Check sheet for the modelled part. Datum: model origin and axes. Units: mm. Face numbers are marked on the shaded views. A direction names the side the tool comes from. Round coordinates to 2 decimals unless told otherwise and drop trailing zeros. Write each loop counter-clockwise with the first axis right and the second up, starting at its lowest first coordinate (ties: lowest second). Pieces come first, ordered by that corner, then holes. Notation, with made-up numbers: (54.25, -16.5) - (106.25, -16.5) arc R6 ccw to (106.25, -9.5) - close; hole circle Ø8 at (44, 13). An arc over 180 degrees is marked (long way). Answer as a JSON object with one key per item and string values. Group by question number.
Item 1: Thickness scan on line 1 (X direction, y = -5.75, z = 55); line 2 (X direction, y = -2.75, z = 22); line 3 (Z direction, x = 14.5, y = -5.25). Record the ranges inside material, lowest first.
Item 2: Set-up check for the marked faces 5, 6 and 7: record each of +Z, -Z, +X, -X, +Y, -Y from which the full face is reachable in a straight line by a thin tool's end or side.
Item 3: Sectioned sample at D-D on y = -2.25. Count the separate pieces of the cut face and the enclosed holes in it, plus the area to 3 significant figures.
Item 4: Sectioned sample at C-C on y = -9.25. Record the boundary of the cut face in (x, z).
Item 5: Sectioned sample at A-A on x = 35. Record the boundary of the cut face in (y, z).
Item 6: Sectioned sample at B-B on z = 18.5. Record the boundary of the cut face in (x, y).
Item 7: Release check for a two-part mould opening along X. For the marked faces 1, 2, 3 and 4 record: pulls with the +X half, pulls with the -X half, needs draft (parallel to the pull), parting line crosses it, or undercut.
Item 8: Gauge pin test, flat ends, axial feed: P1, Ø1.2, axis at y = -4, z = 53.5, coming from the +X side; P2, Ø3, axis at y = -4.5, z = 53, coming from the +X side; P3, Ø4.5, axis at y = -5.5, z = 54, coming from the +X side. Record the tip position at first contact, or that the pin passes through.
```python
from build123d import *

# Parameters (mm, degrees)
F0_W     = 65
F0_H     = 65
F1_DEPTH = 8
F2_W     = 65
F2_H     = 65
F3_DEPTH = 3
F5_DEPTH = 11.001
F7_DEPTH = 11.001
F9_DEPTH = 8
F10_R    = 1


with BuildPart() as f1:
    # F0 (on Front) → F1 (new body)
    with BuildSketch(Plane.XZ):
        with Locations((28.5, 28)):
            Rectangle(F0_W, F0_H)
        Polygon((12, 0), (0, 0), (0, 56), (12, 56), (12, 52), (15, 52), (15, 56), (27, 56), (27, 52), (30, 52), (30, 56), (42, 56), (42, 52), (45, 52), (45, 56), (57, 56), (57, 0), (45, 0), (45, 4), (42, 4), (42, 0), (30, 0), (30, 4), (27, 4), (27, 0), (15, 0), (15, 4), (12, 4), align=None, mode=Mode.SUBTRACT)
    extrude(amount=F1_DEPTH)

    # F2 (on face) → F3 (join)
    with BuildSketch(Plane.XZ.offset(8)):
        with Locations((28.5, 28)):
            Rectangle(F2_W, F2_H)
        Polygon((12, 4), (12, 0), (0, 0), (0, 56), (12, 56), (12, 52), (15, 52), (15, 56), (27, 56), (27, 52), (30, 52), (30, 56), (42, 56), (42, 52), (45, 52), (45, 56), (57, 56), (57, 0), (45, 0), (45, 4), (42, 4), (42, 0), (30, 0), (30, 4), (27, 4), (27, 0), (15, 0), (15, 4), align=None, mode=Mode.SUBTRACT)
        Polygon((0, 0), (12, 0), (12, 4), (15, 4), (15, 0), (27, 0), (27, 4), (30, 4), (30, 0), (42, 0), (42, 4), (45, 4), (45, 0), (57, 0), (57, 56), (45, 56), (45, 52), (42, 52), (42, 56), (30, 56), (30, 52), (27, 52), (27, 56), (15, 56), (15, 52), (12, 52), (12, 56), (0, 56), align=None)
    extrude(amount=F3_DEPTH)

    # F4 (on face) → F5 (cut, through all)
    with BuildSketch(Plane.XZ.offset(11)):
        with BuildLine():
            Line((9.5, 4), (47.5, 4))
            ThreePointArc((47.5, 4), (51.0355339059, 5.4644660941), (52.5, 9))
            Line((52.5, 9), (52.5, 47))
            ThreePointArc((52.5, 47), (51.0355339059, 50.5355339059), (47.5, 52))
            Line((47.5, 52), (9.5, 52))
            ThreePointArc((9.5, 52), (5.9644660941, 50.5355339059), (4.5, 47))
            Line((4.5, 47), (4.5, 9))
            ThreePointArc((4.5, 9), (5.9644660941, 5.4644660941), (9.5, 4))
        make_face()
    extrude(amount=-F5_DEPTH, mode=Mode.SUBTRACT)

    # F6 (on face) → F7 (cut, through all)
    with BuildSketch(Plane.XZ.offset(11)):
        with BuildLine():
            ThreePointArc((-4, 50.8869504303), (0.3925054478, 56.1074945522), (5.6130495697, 60.5))
            Line((5.6130495697, 60.5), (-4, 60.5))
            Line((-4, 60.5), (-4, 50.8869504303))
        make_face()
        with BuildLine():
            Line((61, 60.5), (51.3869504303, 60.5))
            ThreePointArc((51.3869504303, 60.5), (56.6074945522, 56.1074945522), (61, 50.8869504303))
            Line((61, 50.8869504303), (61, 60.5))
        make_face()
        with BuildLine():
            Line((61, -4.5), (61, 5.1130495697))
            ThreePointArc((61, 5.1130495697), (56.6074945522, -0.1074945522), (51.3869504303, -4.5))
            Line((51.3869504303, -4.5), (61, -4.5))
        make_face()
        with BuildLine():
            ThreePointArc((5.6130495697, -4.5), (0.3925054478, -0.1074945522), (-4, 5.1130495697))
            Line((-4, 5.1130495697), (-4, -4.5))
            Line((-4, -4.5), (5.6130495697, -4.5))
        make_face()
    extrude(amount=-F7_DEPTH, mode=Mode.SUBTRACT)

    # F8 (on face) → F9 (cut)
    with BuildSketch(Plane(origin=(0, 0, 0), x_dir=(-1, 0, 0), z_dir=(0, 1, 0))):
        with BuildLine():
            ThreePointArc((-54.9136378655, 57.7049193689), (-55.6366618004, 59.0201509297), (-55.8869504303, 60.5))
            Line((-55.8869504303, 60.5), (-61, 60.5))
            Line((-61, 60.5), (-62.4552159954, 54.6130084653))
            ThreePointArc((-62.4552159954, 54.6130084653), (-58.7438875569, 54.1901486861), (-56.9998547435, 50.8869504303))
            Line((-56.9998547435, 50.8869504303), (-51.3869504303, 50.8869504303))
            Line((-51.3869504303, 50.8869504303), (-51.3869504303, 56))
            Line((-51.3869504303, 56), (-56.7145795645, 56))
            ThreePointArc((-56.7145795645, 56), (-55.8274078977, 56.866507887), (-54.9136378655, 57.7049193689))
        make_face()
        with BuildLine():
            ThreePointArc((-51.3869504303, 56), (-53.3455388455, 56.4485889594), (-54.9136378655, 57.7049193689))
            ThreePointArc((-54.9136378655, 57.7049193689), (-55.8274078977, 56.866507887), (-56.7145795645, 56))
            Line((-56.7145795645, 56), (-51.3869504303, 56))
        make_face()
        with BuildLine():
            ThreePointArc((-0.2854204355, 56), (-1.1725921023, 56.866507887), (-2.0863621345, 57.7049193689))
            ThreePointArc((-2.0863621345, 57.7049193689), (-3.6544611545, 56.4485889594), (-5.6130495697, 56))
            Line((-5.6130495697, 56), (-0.2854204355, 56))
        make_face()
        with BuildLine():
            ThreePointArc((-1.1130495697, 60.5), (-1.3633381996, 59.0201509297), (-2.0863621345, 57.7049193689))
            ThreePointArc((-2.0863621345, 57.7049193689), (-1.1725921023, 56.866507887), (-0.2854204355, 56))
            Line((-0.2854204355, 56), (-5.6130495697, 56))
            Line((-5.6130495697, 56), (-5.6130495697, 50.8869504303))
            Line((-5.6130495697, 50.8869504303), (-0.0001452565, 50.8869504303))
            ThreePointArc((-0.0001452565, 50.8869504303), (1.7438875569, 54.1901486861), (5.4552159954, 54.6130084653))
            Line((5.4552159954, 54.6130084653), (4, 60.5))
            Line((4, 60.5), (-1.1130495697, 60.5))
        make_face()
        with BuildLine():
            Line((-5.6130495697, 5.1130495697), (-5.6130495697, 0))
            ThreePointArc((-5.6130495697, 0), (-2.4310690543, -1.3180194847), (-1.1130495697, -4.5))
            Line((-1.1130495697, -4.5), (4, -4.5))
            Line((4, -4.5), (5.4552159954, 1.3869915347))
            ThreePointArc((5.4552159954, 1.3869915347), (1.7438875569, 1.8098513139), (-0.0001452565, 5.1130495697))
            Line((-0.0001452565, 5.1130495697), (-5.6130495697, 5.1130495697))
        make_face()
        with BuildLine():
            ThreePointArc((-56.9998547435, 5.1130495697), (-58.7438875569, 1.8098513139), (-62.4552159954, 1.3869915347))
            Line((-62.4552159954, 1.3869915347), (-61, -4.5))
            Line((-61, -4.5), (-55.8869504303, -4.5))
            ThreePointArc((-55.8869504303, -4.5), (-54.5689309457, -1.3180194847), (-51.3869504303, 0))
            Line((-51.3869504303, 0), (-51.3869504303, 5.1130495697))
            Line((-51.3869504303, 5.1130495697), (-56.9998547435, 5.1130495697))
        make_face()
    extrude(amount=-F9_DEPTH, mode=Mode.SUBTRACT)

    # F10
    f10_edges = [f1.edges().sort_by_distance(p)[0] for p in [
        (48.193475, 0, 56),
        (45, 0, 54),
        (53.345539, 0, 56.448589),
        (43.5, 0, 52),
        (42, 0, 54),
        (36, 0, 56),
        (30, 0, 54),
        (28.5, 0, 52),
        (27, 0, 54),
        (21, 0, 56),
        (15, 0, 54),
        (13.5, 0, 52),
        (12, 0, 54),
        (8.806525, 0, 56),
        (57, 0, 28),
        (57.411614, 0, 52.654617),
        (57.411614, 0, 3.345383),
        (53.345539, 0, -0.448589),
        (48.193475, 0, 0),
        (45, 0, 2),
        (43.5, 0, 4),
        (42, 0, 2),
        (36, 0, 0),
        (30, 0, 2),
        (28.5, 0, 4),
        (27, 0, 2),
        (21, 0, 0),
        (15, 0, 2),
        (12, 0, 2),
        (8.806525, 0, 0),
        (0, 0, 28),
        (-0.411614, 0, 3.345383),
        (-0.411614, 0, 52.654617),
        (3.654461, 0, 56.448589),
    ]]
    fillet(f10_edges, radius=F10_R)


solid = f1.part
```
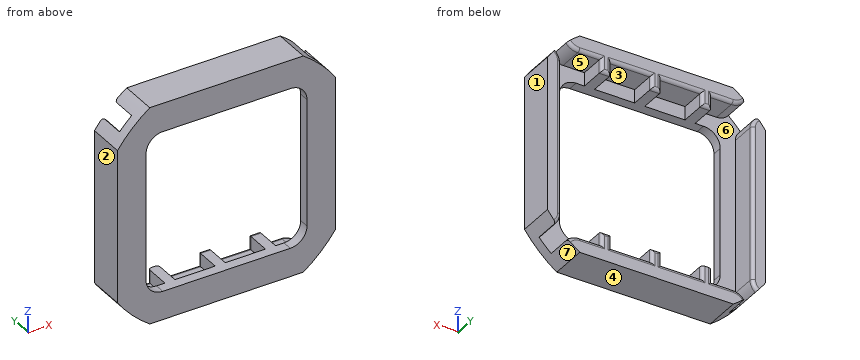
Completed:
{
 "1": {"line 1": "12 to 15, 27 to 30, 42 to 45", "line 2": "-4 to 0, 57 to 61", "line 3": "-4.5 to 4, 52 to 60.5"},
 "2": {"face 5": "+X, +Y", "face 6": "+Y", "face 7": "-Z, +X, +Y, -Y"},
 "3": {"separate pieces": "4", "enclosed holes": "0", "area": "917 mm²"},
 "4": {"outline": "(-4, 5.11) arc R39.75 ccw to (5.61, -4.5) - (51.39, -4.5) arc R39.75 ccw to (61, 5.11) - (61, 50.89) arc R39.75 ccw to (51.39, 60.5) - (5.61, 60.5) arc R39.75 ccw to (-4, 50.89) - close; hole (4.5, 9) arc R5 ccw to (9.5, 4) - (47.5, 4) arc R5 ccw to (52.5, 9) - (52.5, 47) arc R5 ccw to (47.5, 52) - (9.5, 52) arc R5 ccw to (4.5, 47) - close"},
 "5": {"outline": "(-11, -4.5) - (0, -4.5) - (0, -1) arc R1 ccw to (-1, 0) - (-8, 0) - (-8, 4) - (-11, 4) - close; (-11, 52) - (-8, 52) - (-8, 56) - (-1, 56) arc R1 ccw to (0, 57) - (0, 60.5) - (-11, 60.5) - close"},
 "6": {"outline": "(-4, -11) - (4.5, -11) - (4.5, -8) - (0, -8) - (0, -1) arc R1 ccw to (-1, 0) - (-4, 0) - close; (52.5, -11) - (61, -11) - (61, 0) - (58, 0) arc R1 ccw to (57, -1) - (57, -8) - (52.5, -8) - close"},
 "7": {"face 1": "pulls with the +X half", "face 2": "pulls with the -X half", "face 3": "undercut", "face 4": "needs draft"},
 "8": {"P1": "x = 59.48", "P2": "x = 60.56", "P3": "x = 60.37"}
}
